Check sheet for the modelled part. Datum: model origin and axes. Units: mm. Give positions to 0.01 mm unless a question says otherwise; leave off trailing zeros. Write each loop counter-clockwise with the first axis right and the second up, starting at its lowest first coordinate (ties: lowest second). Pieces come first, ordered by that corner, then holes. Notation, with made-up numbers: M -20.75,9.5 L 20.25,9.5 A23 ccw 20.25,45.5 Z; hole C 84,36 d6. An arc over 180 degrees is marked long. Write item = value, one per line. Start each with the question number.
1) Sectioned sample at A-A, the plane z = 23.5. Record the cut outline in (x, y).
2) Gauge pin test, flat ends, axial feed: pin 1 (0.5 mm diameter, centred on y = 0.5, z = 23.5, fed in from +X); pin 2 (4 mm diameter, centred on x = -17.96, z = -17.96, fed in from -Y); pin 3 (0.5 mm diameter, centred on x = 17.5, y = 0.5, fed in from +Z). Record the tip position at first contact, or that the pin passes through.
3) Sectioned sample at B-B, the plane y = 0.5. Count the separate pieces of the cut face and the enclosed holes in it, then the cut area to 3 significant figures.
4) Scan lines: L1, parallel to X at y = 0.65, z = -20; L2, parallel to Z at x = 19, y = 0.05; L3, parallel to Z at x = -16.5, y = 0.1. Record each from-to range of solid material in increasing order.
5) Sectioned sample at C-C, the plane x = 6. Record the cut outline in (y, z) (3 decimals), then the cut area to 3 significant figures.
from build123d import *

# Parameters (mm, degrees)
SKETCH1_R           = 2.25
BOSS_EXTRUDE2_DEPTH = 1


with BuildPart() as part:
    # Sketch1 → Boss-Extrude2 (new body)
    with BuildSketch(Plane(origin=(0, 0, 0), x_dir=(1, 0, 0), z_dir=(0, 1, 0))):
        with BuildLine():
            Line((-17.330956316, -5.08), (-18.669, -5.08))
            ThreePointArc((-18.669, -5.08), (-19.207815367, -4.856815367), (-19.431, -4.318))
            Line((-19.431, -4.318), (-19.431, 4.318))
            ThreePointArc((-19.431, 4.318), (-19.207815367, 4.856815367), (-18.669, 5.08))
            Line((-18.669, 5.08), (-17.330956316, 5.08))
            ThreePointArc((-17.330956316, 5.08), (-16.732344988, 5.370503999), (-16.590161442, 6.020513179))
            ThreePointArc((-16.590161442, 6.020513179), (-18.359695736, 11.0243031), (-21.119367367, 15.557886415))
            ThreePointArc((-21.119367367, 15.557886415), (-21.028176895, 20.478529347), (-16.219689319, 21.527094936))
            ThreePointArc((-16.219689319, 21.527094936), (-14.791805557, 20.867380989), (-13.337157819, 20.268987731))
            ThreePointArc((-13.337157819, 20.268987731), (-10.39690266, 20.611451573), (-9.017, 23.230277748))
            Line((-9.017, 23.230277748), (-9.017, 23.241))
            ThreePointArc((-9.017, 23.241), (-8.942605122, 23.420605122), (-8.763, 23.495))
            Line((-8.763, 23.495), (8.763, 23.495))
            ThreePointArc((8.763, 23.495), (8.942605122, 23.420605122), (9.017, 23.241))
            Line((9.017, 23.241), (9.017, 23.230277748))
            ThreePointArc((9.017, 23.230277748), (10.39690266, 20.611451573), (13.337157819, 20.268987731))
            ThreePointArc((13.337157819, 20.268987731), (14.791805557, 20.867380989), (16.219689319, 21.527094936))
            ThreePointArc((16.219689319, 21.527094936), (21.028176895, 20.478529347), (21.119367367, 15.557886415))
            ThreePointArc((21.119367367, 15.557886415), (18.359695736, 11.0243031), (16.590161442, 6.020513179))
            ThreePointArc((16.590161442, 6.020513179), (16.732344988, 5.370503999), (17.330956316, 5.08))
            Line((17.330956316, 5.08), (18.669, 5.08))
            ThreePointArc((18.669, 5.08), (19.207815367, 4.856815367), (19.431, 4.318))
            Line((19.431, 4.318), (19.431, -4.318))
            ThreePointArc((19.431, -4.318), (19.207815367, -4.856815367), (18.669, -5.08))
            Line((18.669, -5.08), (17.330956316, -5.08))
            ThreePointArc((17.330956316, -5.08), (16.732344988, -5.370503999), (16.590161442, -6.020513179))
            ThreePointArc((16.590161442, -6.020513179), (18.359695736, -11.0243031), (21.119367367, -15.557886415))
            ThreePointArc((21.119367367, -15.557886415), (21.028176895, -20.478529347), (16.219689319, -21.527094936))
            ThreePointArc((16.219689319, -21.527094936), (11.752669663, -19.697385754), (7.085365092, -18.465164862))
            ThreePointArc((7.085365092, -18.465164862), (4.458452771, -19.130602125), (3.302, -21.581335094))
            Line((3.302, -21.581335094), (3.302, -25.4))
            ThreePointArc((3.302, -25.4), (3.116012806, -25.849012806), (2.667, -26.035))
            Line((2.667, -26.035), (-2.667, -26.035))
            ThreePointArc((-2.667, -26.035), (-3.116012806, -25.849012806), (-3.302, -25.4))
            Line((-3.302, -25.4), (-3.302, -21.581335094))
            ThreePointArc((-3.302, -21.581335094), (-4.458452771, -19.130602125), (-7.085365092, -18.465164862))
            ThreePointArc((-7.085365092, -18.465164862), (-11.752669663, -19.697385754), (-16.219689319, -21.527094936))
            ThreePointArc((-16.219689319, -21.527094936), (-21.028176895, -20.478529347), (-21.119367367, -15.557886415))
            ThreePointArc((-21.119367367, -15.557886415), (-18.359695736, -11.0243031), (-16.590161442, -6.020513179))
            ThreePointArc((-16.590161442, -6.020513179), (-16.732344988, -5.370503999), (-17.330956316, -5.08))
        make_face()
        with Locations((-17.960512242, -17.960512242)):
            Circle(SKETCH1_R, mode=Mode.SUBTRACT)
        with Locations((17.960512242, -17.960512242)):
            Circle(SKETCH1_R, mode=Mode.SUBTRACT)
        with Locations((17.960512242, 17.960512242)):
            Circle(SKETCH1_R, mode=Mode.SUBTRACT)
        with Locations((-17.960512242, 17.960512242)):
            Circle(SKETCH1_R, mode=Mode.SUBTRACT)
    extrude(amount=BOSS_EXTRUDE2_DEPTH)


solid = part.part
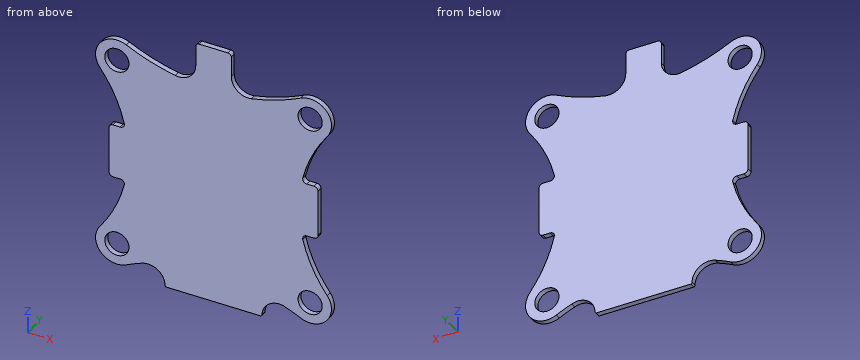
Data:
q1.outline = M -3.3,0 L 3.3,0 L 3.3,1 L -3.3,1 Z
q2.pin_1 = 3.3
q2.pin_2 = through
q2.pin_3 = 21.92
q3.separate_pieces = 1
q3.enclosed_holes = 4
q3.area = 1,620 mm2
q4.L1 = -21.37 to -18.91, -17.01 to 17.01, 18.91 to 21.37
q4.L2 = -21.79 to -19.96, -15.97 to -12.28, -5 to 5, 12.28 to 15.97, 19.96 to 21.79
q4.L3 = -21.65 to -19.67, -16.25 to 16.25, 19.67 to 21.65
q5.outline = M 0,-23.495 L 1,-23.495 L 1,18.442 L 0,18.442 Z
q5.area = 41.9 mm2
